```python
from build123d import *

# Parameters (mm, degrees)
SKETCH1_W           = 88.9
SKETCH1_H           = 25.4
BOSS_EXTRUDE1_DEPTH = 25.4
SKETCH2_RX          = 25.4
SKETCH2_RY          = 15.24
CUT_EXTRUDE1_DEPTH  = 58.15
FILLET1_R           = 2.54
SKETCH5_R           = 3.81
CUT_EXTRUDE2_DEPTH  = 53.747061686
FILLET2_R           = 22.86


with BuildPart() as part:
    # Sketch1 → Boss-Extrude1 (new body)
    with BuildSketch(Plane(origin=(0, 0, 0), x_dir=(1, 0, 0), z_dir=(0, 1, 0))):
        Rectangle(SKETCH1_W, SKETCH1_H)
    extrude(amount=BOSS_EXTRUDE1_DEPTH)

    # Sketch2 → Cut-Extrude1 (cut, through all)
    with BuildSketch(Plane.XY.offset(12.7)):
        with Locations(Location((-12.7, 25.4), (0, 0, 180))):
            Ellipse(SKETCH2_RX, SKETCH2_RY)
    extrude(amount=-CUT_EXTRUDE1_DEPTH, mode=Mode.SUBTRACT)

    # Fillet1
    fillet1_edges = [part.edges().sort_by_distance(p)[0] for p in [
        (-38.1, 25.4, 0),
    ]]
    fillet(fillet1_edges, radius=FILLET1_R)

    # Sketch5 → Cut-Extrude2 (cut, through all)
    with BuildSketch(Plane(origin=(0, 25.4, 0), x_dir=(1, 0, 0), z_dir=(0, 1, 0))):
        with Locations(Location((34.29, 6.35, 0), (0, 0, 270))):
            Circle(SKETCH5_R)
        with Locations(Location((34.29, -6.35, 0), (0, 0, 270))):
            Circle(SKETCH5_R)
    extrude(amount=-CUT_EXTRUDE2_DEPTH, mode=Mode.SUBTRACT)

    # Fillet2
    fillet2_edges = [part.edges().sort_by_distance(p)[0] for p in [
        (-44.45, 0, 0),
    ]]
    fillet(fillet2_edges, radius=FILLET2_R)


solid = part.part
```
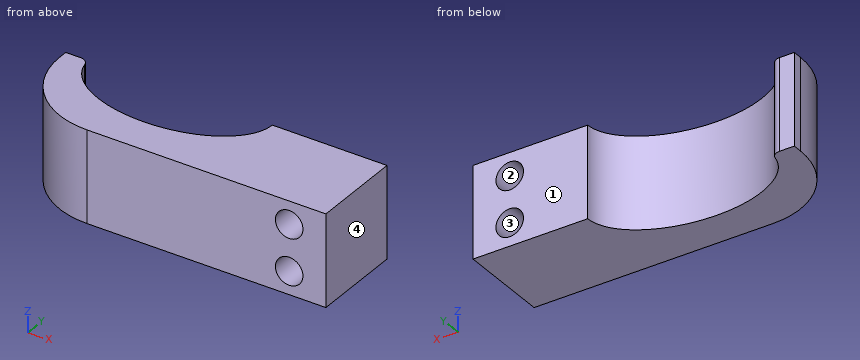
Input: part model. Units: mm. Frame: model coordinates. Face numbers are marked on the shaded views. Round coordinates to 2 decimals unless told otherwise and drop trailing zeros. Loops run counter-clockwise (first coordinate to the right, second up) from the corner with the lowest first, then second, coordinate; pieces in that order, holes last. Notation, with made-up numbers: M 51,-12.5 L 93,-12.5 A19 ccw 93,5.5 Z; hole C -2,41.25 d3. An arc over 180 degrees is marked long. Answer in a Markdown table with one row per item. Add a question column.
1. Section C-C (y = 7.5). Output: boundary loops of the cut face in (x, z).
2. Section A-A (x = 37). Output: boundary loops of the cut face in (y, z), and give its area (3 significant figures).
3. Section B-B (y = 17.5). Give the number of separate pieces and of enclosed holes in the cut face, and give its area (3 significant figures).
4. Mould query, pull axis X, two halves, no side actions, for the marked faces 1, 2, 3 and 4. Classes: released by +X, released by -X, zero draft, split by the parting line, or undercut.
5. Contact query for flat-ended pins moving along their axis: pin 1 (8 mm diameter, centred on x = -19, y = 16.5, fed in from -Z); pin 2 (12 mm diameter, centred on y = 10.5, z = -9.5, fed in from -X); pin 3 (1.5 mm diameter, centred on y = 3.5, z = 5, fed in from -X). Output: stop coordinate, or through.
6. Ray query, probe 1 along X at (y, z) = (17.25, 9.5); probe 2 along X at (y, z) = (13.25, 6.35); probe 3 along Z at (x, y) = (36, 1.5). Return the intervals inside material, ascending.
Values follow:
| question | item | result |
|---|---|---|
| 1 | outline | M -38.52,-12.7 L 44.45,-12.7 L 44.45,12.7 L -38.52,12.7 Z; hole C 34.29,-6.35 d7.62; hole C 34.29,6.35 d7.62 |
| 2 | outline | M 0,-12.7 L 25.4,-12.7 L 25.4,-9.03 L 0,-9.03 Z; M 0,-3.67 L 25.4,-3.67 L 25.4,3.67 L 0,3.67 Z; M 0,9.03 L 25.4,9.03 L 25.4,12.7 L 0,12.7 Z |
| 2 | area | 373 mm^2 |
| 3 | separate pieces | 2 |
| 3 | enclosed holes | 2 |
| 3 | area | 1,050 mm^2 |
| 4 | face 1 | zero draft |
| 4 | face 2 | undercut |
| 4 | face 3 | undercut |
| 4 | face 4 | released by +X |
| 5 | pin 1 | through |
| 5 | pin 2 | x = -43.55 |
| 5 | pin 3 | x = -34.87 |
| 6 | probe 1 | -43.75 to -34.16, 8.76 to 32.15, 36.43 to 44.45 |
| 6 | probe 2 | -42.33 to -28.03, 2.63 to 30.48, 38.1 to 44.45 |
| 6 | probe 3 | -12.7 to -9.75, -2.95 to 2.95, 9.75 to 12.7 |
